The drawing under review shows one solid part. Ordinate dimensions are in mm from its lowest x, y, z. Round coordinates to 2 decimals unless told otherwise and drop trailing zeros. Write each loop counter-clockwise with the first axis right and the second up, starting at its lowest first coordinate (ties: lowest second). Pieces come first, ordered by that corner, then holes. Notation, with made-up numbers: (-39.5, 80) -> (-31.5, 80) arc R12 cw to (-31.5, 90) -> close; hole circle Ø4 at (16.5, 7.25). An arc over 180 degrees is marked (long way). Answer in a Markdown table with one row per item. Add a question column.
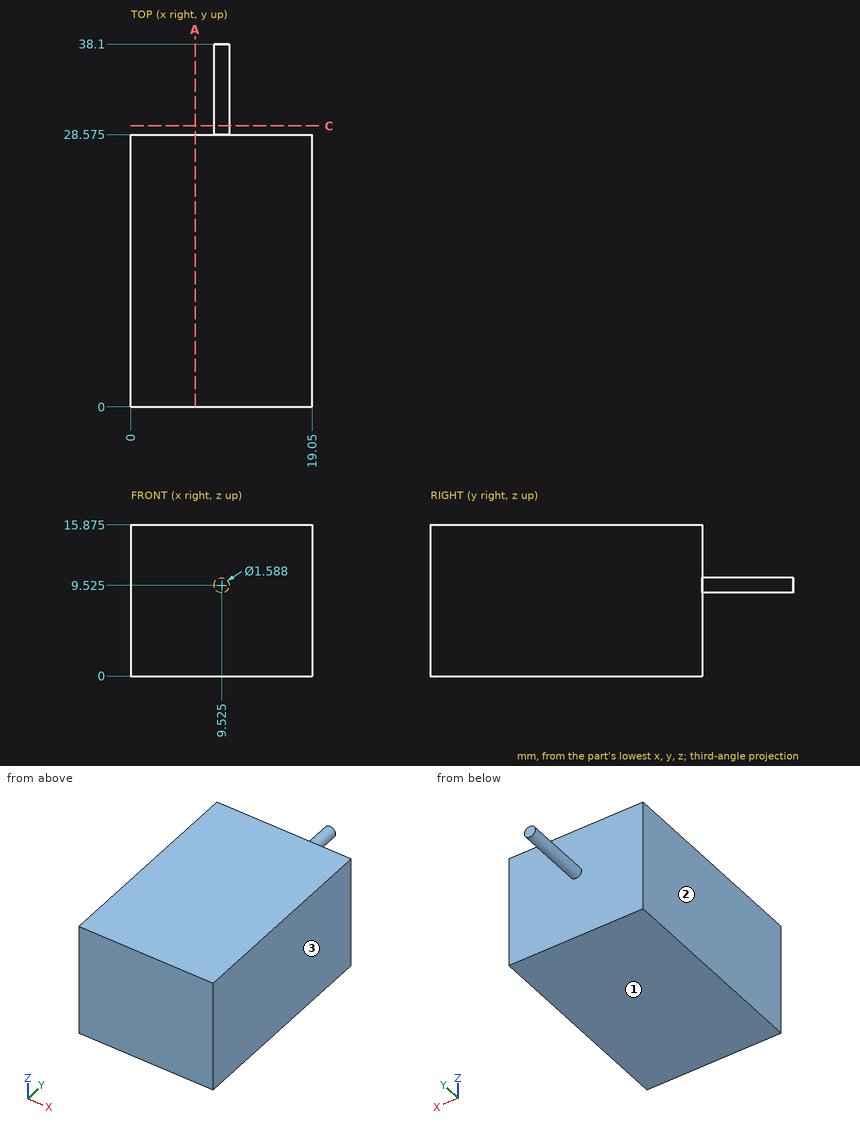
1. For L1, parallel to Y at x = 5, z = 8.75 (1 decimal), list the stretches that pass through material, from the lowest coordinate up.
2. Add section C-C on y = 29.5. Write out the cut boundary in (x, z) (1 decimal).
3. Mouldability with a two-part tool opening along X and no side actions: class the marked faces 1, 2 and 3 as pulls with the +X half, pulls with the -X half, needs draft (parallel to the pull), parting line crosses it, or undercut.
4. Add section A-A on x = 6.75. Write out the cut boundary in (y, z) (1 decimal).
5. Insertion check: pin 1 Ø5 at (x, y) = (13, 34) entering from +Z; pin 2 Ø4 at (x, z) = (6, 7) entering from +Y (1 decimal); pin 3 Ø1 at (y, z) = (32.5, 10) entering from -X. Each pin has a flat end and moves straight along its axis. Give the tip position at first contact, or say it passes through.
Filled in:
| question | item | result |
|---|---|---|
| 1 | L1 | 0 to 28.6 |
| 2 | outline | circle Ø1.6 at (9.5, 9.5) |
| 3 | face 1 | needs draft |
| 3 | face 2 | pulls with the -X half |
| 3 | face 3 | pulls with the +X half |
| 4 | outline | (0, 0) -> (28.6, 0) -> (28.6, 15.9) -> (0, 15.9) -> close |
| 5 | pin 1 | through |
| 5 | pin 2 | y = 28.6 |
| 5 | pin 3 | x = 8.73 |
